The listing builds one solid part. Answer for the finished solid, in the listing's coordinates (mm). A direction names the side the tool comes from. Coordinates: 2 decimals unless noted, no trailing zeros. Write each loop counter-clockwise with the first axis right and the second up, starting at its lowest first coordinate (ties: lowest second). Pieces come first, ordered by that corner, then holes.
Autodesk Fusion 360 part; units mm, degrees
sketch "Sketch1" plane through (0, 0, 0) normal (0, 0, 1) x (1, 0, 0)
  line L0 (0, 0) -> (40, 0)
  line L1 (40, 0) -> (40, 42)
  line L2 (40, 42) -> (0, 42)
  line L3 (0, 42) -> (0, 0)
  dimension "d1" = 40
  dimension "d2" = 42
extrude "Extrude1" add sketch "Sketch1" along normal blind 2.5
sketch "Sketch2" plane through (40, 0, 0) normal (1, 0, 0) x (0, 1, 0)
  line L0 (0, 0) -> (42, 0)
  line L1 (42, 0) -> (42, 2.5)
  line L2 (42, 2.5) -> (0, 2.5)
  line L3 (0, 2.5) -> (0, 0)
  line L4 (3, 2.5) -> (12.5, 2.5)
  line L5 (12.5, 2.5) -> (12.5, 0)
  line L6 (12.5, 0) -> (3, 0)
  line L7 (3, 0) -> (3, 2.5)
  dimension "d5" = 9.5
  dimension "d6" = 3
extrude "Extrude2" add sketch "Sketch2" along normal blind 3 contours L0 L2 L4 L5 L6 L7
sketch "Sketch3" plane through (0, 0, 0) normal (-1, 0, 0) x (0, -1, 0)
  line L0 (-42, 0) -> (0, 0)
  line L1 (0, 0) -> (0, 2.5)
  line L2 (0, 2.5) -> (-42, 2.5)
  line L3 (-42, 2.5) -> (-42, 0)
  line L4 (-3, 2.5) -> (-12.5, 2.5)
  line L5 (-12.5, 2.5) -> (-12.5, 0)
  line L6 (-12.5, 0) -> (-3, 0)
  line L7 (-3, 0) -> (-3, 2.5)
  dimension "d9" = 9.5
  dimension "d10" = 2.5
  dimension "d11" = 3
extrude "Extrude3" add sketch "Sketch3" along normal blind 3 contours L0 L2 L4 L5 L6 L7
sketch "Sketch4" plane through (0, 0, 2.5) normal (0, 0, 1) x (-1, 0, 0)
  line L0 (0, -42) -> (0, -12.5)
  line L1 (0, -12.5) -> (3, -12.5)
  line L2 (3, -12.5) -> (3, -3)
  line L3 (3, -3) -> (0, -3)
  line L4 (0, -3) -> (0, 0)
  line L5 (0, 0) -> (-40, 0)
  line L6 (-40, 0) -> (-40, -3)
  line L7 (-40, -3) -> (-43, -3)
  line L8 (-43, -3) -> (-43, -12.5)
  line L9 (-43, -12.5) -> (-40, -12.5)
  line L10 (-40, -12.5) -> (-40, -42)
  line L11 (-40, -42) -> (0, -42)
  line L12 (-8.5, -39.5) -> (-31.5, -39.5)
  line L13 (-31.5, -39.5) -> (-31.5, -26.5)
  line L14 (-31.5, -26.5) -> (-8.5, -26.5)
  line L15 (-8.5, -26.5) -> (-8.5, -39.5)
  dimension "d14" = 23
  dimension "d15" = 13
  dimension "d16" = 8.5
  dimension "d17" = 14
extrude "Extrude4" cut sketch "Sketch4" against normal blind 3 contours L12 L13 L14 L15
sketch "Sketch5" plane through (0, 0, 2.5) normal (0, 0, 1) x (-1, 0, 0)
  line L0 (-31.5, -39.5) -> (-31.5, -26.5)
  line L1 (-31.5, -26.5) -> (-8.5, -26.5)
  line L2 (-8.5, -26.5) -> (-8.5, -39.5)
  line L3 (-8.5, -39.5) -> (-31.5, -39.5)
  line L4 (0, -42) -> (0, -12.5)
  line L5 (0, -12.5) -> (3, -12.5)
  line L6 (3, -12.5) -> (3, -3)
  line L7 (3, -3) -> (0, -3)
  line L8 (0, -3) -> (0, 0)
  line L9 (0, 0) -> (-40, 0)
  line L10 (-40, 0) -> (-40, -3)
  line L11 (-40, -3) -> (-43, -3)
  line L12 (-43, -3) -> (-43, -12.5)
  line L13 (-43, -12.5) -> (-40, -12.5)
  line L14 (-40, -12.5) -> (-40, -42)
  line L15 (-40, -42) -> (0, -42)
  circle A0 centre (-6.25, -33) radius 1.25
  dimension "d24" = 2.5
  dimension "d25" = 2.25
  dimension "d26" = 6.5
extrude "Extrude5" cut sketch "Sketch5" against normal blind 3 contours A0
sketch "Sketch6" plane through (0, 0, 2.5) normal (0, 0, 1) x (-1, 0, 0)
  circle A0 centre (-6.25, -33) radius 1.25
  line L0 (-31.5, -39.5) -> (-31.5, -26.5)
  line L1 (-31.5, -26.5) -> (-8.5, -26.5)
  line L2 (-8.5, -26.5) -> (-8.5, -39.5)
  line L3 (-8.5, -39.5) -> (-31.5, -39.5)
  line L4 (0, -42) -> (0, -12.5)
  line L5 (0, -12.5) -> (3, -12.5)
  line L6 (3, -12.5) -> (3, -3)
  line L7 (3, -3) -> (0, -3)
  line L8 (0, -3) -> (0, 0)
  line L9 (0, 0) -> (-40, 0)
  line L10 (-40, 0) -> (-40, -3)
  line L11 (-40, -3) -> (-43, -3)
  line L12 (-43, -3) -> (-43, -12.5)
  line L13 (-43, -12.5) -> (-40, -12.5)
  line L14 (-40, -12.5) -> (-40, -42)
  line L15 (-40, -42) -> (0, -42)
  circle A1 centre (-33.75, -33) radius 1.25
  dimension "d29" = 2.5
  dimension "d30" = 2.25
  dimension "d31" = 6.5
extrude "Extrude6" cut sketch "Sketch6" against normal blind 3 contours A1
extrude "Extrude7" add 1 faces at (40, 22.3333, 0.8333) along direction (1, 0, 0) blind 0.5
extrude "Extrude8" add 1 faces at (40, 2, 1.6667) along direction (1, 0, 0) blind 0.5
extrude "Extrude9" add 1 faces at (0, 32.1667, 0.8333) along direction (-1, 0, 0) blind 0.5
extrude "Extrude10" add 1 faces at (0, 1, 1.6667) along direction (-1, 0, 0) blind 0.5
extrude "Extrude11" add 1 faces at (-3, 9.3333, 1.6667) along direction (-1, 0, 0) blind 0.5
extrude "Extrude12" add 1 faces at (43, 6.1667, 1.6667) along direction (1, 0, 0) blind 0.5
fillet "Fillet3" radius 5 1 edges at (-0.5, 42, 1.25)
fillet "Fillet4" radius 5 1 edges at (40.5, 42, 1.25)
(1) Section A-A, the plane x = 30 is taken. Write down the section's boundary in (y, z), plus the area to 3 significant figures.
(2) Section D-D, the plane x = 6.25 is taken. Write down the section's boundary in (y, z).
(3) Section C-C, the plane y = 33 is taken. Write down the section's boundary in (x, z).
(4) Section B-B, the plane z = 1.6 is taken. Write down the section's boundary in (x, y), plus the area to 3 significant figures.
(5) Find the intervals of material crossed by probe 1 along X at (y, z) = (33, 0.95); probe 2 along Y at (x, z) = (33.75, 1.95); probe 3 along Y at (x, z) = (19.5, 2.1), in increasing order.
(6) Each of these flat-tipped pins is pushed along its axis until it touches: pin 1 (1.2 mm diameter, centred on y = 30.5, z = 1.5, fed in from -X); pin 2 (0.8 mm diameter, centred on x = 42.5, z = 1, fed in from +Y). Where does it stop, or does it pass through?
(7) Which of the six approach directions +Z, -Z, +X, -X, +Y, -Y give full straight-line access (tool end or side, diameter ignored) to faces 1 (the flat face through (-2, 12.5, 1)), 2 (the flat face through (-2, 3, 1)), 3 (the flat face through (31.5, 33, 1)), 4 (the flat face through (42, 3, 1))?
(8) For a pull along X with two mould halves and no side action, classify faces 5 (the flat face through (40.5, 1, 1)), 6 (the cylindrical face through (7.5, 32.95, 1.27)), 7 (the flat face through (20, 16, 0)) as pulls with the +X half, pulls with the -X half, needs draft (parallel to the pull), parting line crosses it, or undercut.
Solution:
1. outline: (0, 0) - (26.5, 0) - (26.5, 2.5) - (0, 2.5) - close; (39.5, 0) - (42, 0) - (42, 2.5) - (39.5, 2.5) - close
1. area: 72.5 mm2
2. outline: (0, 0) - (31.75, 0) - (31.75, 2.5) - (0, 2.5) - close; (34.25, 0) - (42, 0) - (42, 2.5) - (34.25, 2.5) - close
3. outline: (-0.5, 0) - (5, 0) - (5, 2.5) - (-0.5, 2.5) - close; (7.5, 0) - (8.5, 0) - (8.5, 2.5) - (7.5, 2.5) - close; (31.5, 0) - (32.5, 0) - (32.5, 2.5) - (31.5, 2.5) - close; (35, 0) - (40.5, 0) - (40.5, 2.5) - (35, 2.5) - close
4. outline: (-3.5, 3) - (-0.5, 3) - (-0.5, 0) - (40.5, 0) - (40.5, 3) - (43.5, 3) - (43.5, 12.5) - (40.5, 12.5) - (40.5, 37) arc R5 ccw to (35.5, 42) - (4.5, 42) arc R5 ccw to (-0.5, 37) - (-0.5, 12.5) - (-3.5, 12.5) - close; hole circle Ø2.5 at (6.25, 33); hole (8.5, 26.5) - (31.5, 26.5) - (31.5, 39.5) - (8.5, 39.5) - close; hole circle Ø2.5 at (33.75, 33)
4. area: 1,460 mm2
5. probe 1: x = -0.5 to 5, 7.5 to 8.5, 31.5 to 32.5, 35 to 40.5
5. probe 2: y = 0 to 31.75, 34.25 to 42
5. probe 3: y = 0 to 26.5, 39.5 to 42
6. pin 1: stops at x = -0.5
6. pin 2: stops at y = 12.5
7. face 1: +Z, -Z, -X, +Y
7. face 2: +Z, -Z, -X, -Y
7. face 3: +Z, -Z
7. face 4: +Z, -Z, +X, -Y
8. face 5: pulls with the +X half
8. face 6: undercut
8. face 7: needs draft
